Check sheet for the modelled part. Datum: model origin and axes. Units: mm. Face numbers are marked on the shaded views. A direction names the side the tool comes from. Round coordinates to 2 decimals unless told otherwise and drop trailing zeros. Order: outer loops, then holes, each group sorted by start corner. A loop starts at its lowest first (then second) coordinate and runs counter-clockwise, first axis right, second up.
Q1. Cross-section at C-C on y = -11. Record the cut outline in (x, z), then the cut area to 3 significant figures.
Q2. Depth check by flat-ended pin: P1, Ø3, axis at x = -7.5, y = -12, coming from the +Z side; P2, Ø13, axis at x = 0, y = 0, coming from the +Z side; P3, Ø1, axis at x = 5.5, z = 0.5, coming from the -Y side; P4, Ø6, axis at x = 9.5, z = 3.5, coming from the -Y side. Enter the tip coordinate at first touch or a pass-through.
Q3. Cross-section at D-D on x = -3.5. Record the cut outline in (y, z), then the cut area to 3 significant figures.
Q4. Mould release check, pull along X, two halves, no side actions. Record for the marked faces 3, 4 and 5: +X half, -X half, draft (parallel to the pull), parting line (faces both ways), or undercut.
Q5. Cross-section at B-B on y = 0. Record the cut outline in (x, z), then the cut area to 3 significant figures.
Q6. Scan lines: probe 1 along X at (y, z) = (0, 0.85); probe 2 along Y at (x, z) = (0, 5.5); probe 3 along Y at (x, z) = (0, 0.6). Record each from-to range of solid material in increasing order.
Q7. Set-up check for the marked faces 1 and 2: record each of +Z, -Z, +X, -X, +Y, -Y from which the full face is reachable in a straight line by a thin tool's end or side.
Q8. Cross-section at A-A on x = 0. Record the cut outline in (y, z), then the cut area to 3 significant figures.
from build123d import *

# Parameters (mm, degrees)
F0_R     = 15.9
F0_R_2   = 4
F1_DEPTH = 10
F2_T     = -1.2
F3_DEPTH = 10.001
F4_DEPTH = 0.8
F5_W     = 2
F5_H     = 3.5
F6_DEPTH = 10.801


# Not quite as in the source:
# - a feature names something its author has since deleted; it is built from what else it names


with BuildPart() as f1:
    # F0 (on Top) → F1 (new body)
    with BuildSketch(Plane.XY):
        Circle(F0_R)
        Circle(F0_R_2, mode=Mode.SUBTRACT)
        Circle(F0_R_2)
    extrude(amount=F1_DEPTH)

    # F2
    f2_openings = [f1.faces().sort_by_distance(p)[0] for p in [
        (0, 0, 10),
    ]]
    offset(amount=F2_T, openings=f2_openings)

    # F0 (on Top) → F3 (cut, through all)
    with BuildSketch(Plane.XY):
        Circle(F0_R_2)
    extrude(amount=F3_DEPTH, mode=Mode.SUBTRACT)

    # F0 (on Top) → F4 (join)
    with BuildSketch(Plane.XY):
        Circle(F0_R)
        Circle(F0_R_2, mode=Mode.SUBTRACT)
    extrude(amount=-F4_DEPTH)

    # F5 (on face) → F6 (cut, through all)
    with BuildSketch(Plane(origin=(0, 0, -0.8), x_dir=(1, 0, 0), z_dir=(0, 0, -1))):
        with Locations((5.9, 0)):
            Rectangle(F5_W, F5_H)
        with BuildLine():
            ThreePointArc((15.9, 0), (15.4176846511, 3.8865151486), (14, 7.5372408745))
            Line((14, 7.5372408745), (14, -7.5372408745))
            ThreePointArc((14, -7.5372408745), (15.4176846511, -3.8865151486), (15.9, 0))
        make_face()
    extrude(amount=-F6_DEPTH, mode=Mode.SUBTRACT)


solid = f1.part
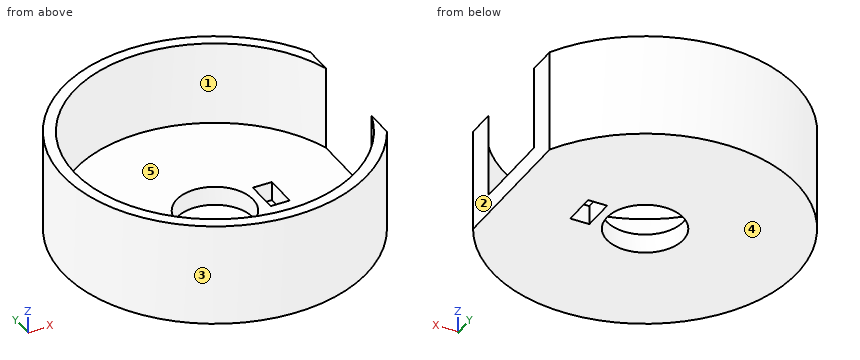
Results found:
1. outline: (-11.48, -0.8) - (11.48, -0.8) - (11.48, 10) - (9.75, 10) - (9.75, 1.2) - (-9.75, 1.2) - (-9.75, 10) - (-11.48, 10) - close
1. area: 76.4 mm2
2. P1: stops at z = 10
2. P2: stops at z = 1.2
2. P3: stops at y = -15.09
2. P4: stops at y = -14.51
3. outline: (-15.51, -0.8) - (-1.94, -0.8) - (-1.94, 1.2) - (-14.28, 1.2) - (-14.28, 10) - (-15.51, 10) - close; (1.94, -0.8) - (15.51, -0.8) - (15.51, 10) - (14.28, 10) - (14.28, 1.2) - (1.94, 1.2) - close
3. area: 76.0 mm2
4. face 3: parting line
4. face 4: draft
4. face 5: undercut
5. outline: (-15.9, -0.8) - (-4, -0.8) - (-4, 1.2) - (-14.7, 1.2) - (-14.7, 10) - (-15.9, 10) - close; (4, -0.8) - (4.9, -0.8) - (4.9, 1.2) - (4, 1.2) - close; (6.9, -0.8) - (14, -0.8) - (14, 1.2) - (6.9, 1.2) - close
5. area: 50.4 mm2
6. probe 1: x = -15.9 to -4, 4 to 4.9, 6.9 to 14
6. probe 2: y = -15.9 to -14.7, 14.7 to 15.9
6. probe 3: y = -15.9 to -4, 4 to 15.9
7. face 1: +Z
7. face 2: +Z, -Z, +X, +Y, -Y
8. outline: (-15.9, -0.8) - (-4, -0.8) - (-4, 1.2) - (-14.7, 1.2) - (-14.7, 10) - (-15.9, 10) - close; (4, -0.8) - (15.9, -0.8) - (15.9, 10) - (14.7, 10) - (14.7, 1.2) - (4, 1.2) - close
8. area: 68.7 mm2
